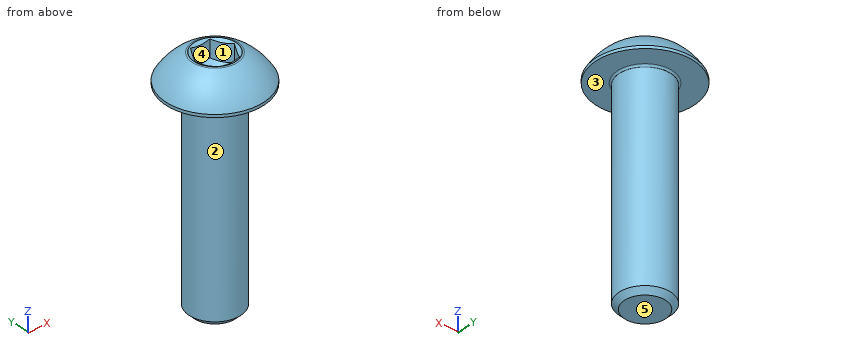
Solid Edge part; units mm, degrees
sketch "Sketch1" plane through (0, 0, 0) normal (0, -1, 0) x (1, 0, 0)
  line L0 (0, -12) -> (1.5, -12)
  line L1 (1.5, -12) -> (1.5, -0.115)
  arc A0 (1.5, -0.105) -> (1.5, -0.115) centre (1.5037, -0.11) ccw
  line L2 (1.5, -0.105) -> (1.5, 0)
  line L3 (1.5, 0) -> (2.85, 0)
  line L4 (2.85, 0) -> (2.85, 0.165)
  arc A1 (1.27, 1.65) -> (2.85, 0.165) centre (-0.3628, -1.6703) cw
  line L5 (0, 1.65) -> (1.27, 1.65)
  dimension "D1" = 1.5
revolve "RevolvedProtrusion1" add sketch "Sketch1" angle 360 about axis through (0, 0, 5) along (0, 0, -1)
sketch "Sketch2" plane through (0, 0, 0) normal (0, -1, 0) x (1, 0, 0)
  line L0 (0, -0.0566) -> (1.1545, 0.61)
  line L1 (1.1545, 0.61) -> (1.1545, 1.65)
  line L2 (1.1545, 1.65) -> (0, 1.65)
revolve "RevolvedCutout1" cut sketch "Sketch2" angle 360 about axis through (0, 0, 5.3) along (0, 0, -1)
sketch "Sketch3" plane through (0, 0, 0) normal (0, 0, -1) x (0, 1, 0)
  arc A0 (-1, 0.577) -> (-1, -0.577) centre (0, 0) ccw
  line L0 (-1, 0.577) -> (-1, -0.577)
extrude "Protrusion1" add sketch "Sketch3" against normal blind 1.65
pattern_circular "Pattern1" count 6 over 360 about axis through (0, 0, 0) along (0, 0, -1) of "Protrusion1"
fillet "Round_1" radius 0.185 1 edges at (-1.27, 0, 1.65)
sketch "Sketch4" plane through (0, 0, 0) normal (0, -1, 0) x (1, 0, 0)
  line L0 (0, 0.9501) -> (1.2122, 1.65)
  line L1 (1.2122, 1.65) -> (0, 1.65)
revolve "RevolvedCutout2" cut sketch "Sketch4" angle 360 about axis through (0, 0, 5.3) along (0, 0, -1)
sketch "Sketch5" plane through (0, 0, 0) normal (0, -1, 0) x (1, 0, 0)
  line L0 (-1.5, 0) -> (-1.5, -0.1)
  line L1 (-1.6, 0) -> (-1.5, 0)
  arc A0 (-1.6, 0) -> (-1.5, -0.1) centre (-1.6, -0.1) cw
revolve "RevolvedProtrusion2" add sketch "Sketch5" angle 360 about axis through (0, 0, -0.5) along (0, 0, 1)
cosmetic_thread "Thread1"
chamfer "Chamfer1" distance 0.3065 angle 45 1 edges at (-1.5, 0, -12)
properties material "Stahl"
Build history of the part. All positions in model axes, mm. Face numbers are marked on the shaded views. A direction names the side the tool comes from. Give positions to 0.01 mm unless a question says otherwise; leave off trailing zeros. Loops run counter-clockwise (first coordinate to the right, second up) from the corner with the lowest first, then second, coordinate; pieces in that order, holes last. Notation, with made-up numbers: (21.5, -25.75) -> (80.5, -25.75) arc R12 ccw to (80.5, -8.75) -> close; hole circle Ø5 at (-13, 32.5). An arc over 180 degrees is marked (long way). One line per question, with ' | ' between items. Start each with the question number.
1) Two-plate mould, pull along X, no slides. Class the marked faces 1, 2 and 3: released by +X, released by -X, zero draft, split by the parting line, or undercut.
2) 3-axis set-ups, long thin cutter, end or side, ignore diameter. For the marked faces 4 and 5: which of +Z, -Z, +X, -X, +Y, -Y reach the whole face in a straight line?
3) Probe L1, parallel to Z at x = 2.45, y = 0.8; L2, parallel to Y at x = -0.1, z = 0.75; L3, parallel to Y at x = 0.7, z = -3.25. List the from-to ranges inside material, lowest first.
4) Cut at A-A (z = -0.25). Give the cut face in (x, y), plus the area to 3 significant figures.
5) Pin check, flat tips, straight feed: pin 1 (1 mm diameter, centred on y = 1.5, z = -2, fed in from +X); pin 2 (0.5 mm diameter, centred on x = 0, z = 1.5, fed in from +Y). Stop position of each tip, or through.
Return value:
1) face 1: undercut | face 2: split by the parting line | face 3: zero draft
2) face 4: +Z | face 5: -Z, +X, -X, +Y, -Y
3) L1: 0 to 0.58 | L2: -2.43 to -1, 1 to 2.43 | L3: -1.33 to 1.33
4) outline: circle Ø3 at (0, 0) | area: 7.07 mm^2
5) pin 1: x = 1.12 | pin 2: y = 1.91
